from build123d import *

# Parameters (mm, degrees)
F1_DEPTH = 90


with BuildPart() as f1:
    # F0 (on Front) → F1 (new body)
    with BuildSketch(Plane.XZ):
        with BuildLine():
            Line((54.3923101205, -6.9459271067), (39.3923101205, -6.9459271067))
            Line((39.3923101205, -6.9459271067), (24.3923101205, -6.9459271067))
            Line((24.3923101205, -6.9459271067), (24.3923101205, -22.9459271067))
            ThreePointArc((24.3923101205, -22.9459271067), (27.0283490898, -29.3098881374), (33.3923101205, -31.9459271067))
            Line((33.3923101205, -31.9459271067), (39.3923101205, -31.9459271067))
            add(Edge.make_bspline(
                [(54.3923101205, -6.9459271067), (54.7600798309, -12.4650411308), (53.5760512989, -19.2747786322), (51.1416965676, -25.5090219107), (47.6191843875, -29.9359194122), (42.847190561, -31.9967957119), (39.3923101205, -31.9459271067)],
                knots=[0, 0, 0, 0, 0.318087546, 0.5385673182, 0.7419978267, 1, 1, 1, 1], degree=3))
        make_face()
        with BuildLine():
            Line((24.3923101205, -6.9459271067), (39.3923101205, -6.9459271067))
            add(Edge.make_bspline(
                [(39.3923101205, -6.9459271067), (34.4260372221, -4.787703976), (28.490868897, -2.8215542068), (10.9690373288, 1.5413653414), (3.5167664753, 1.7551726321), (0, 1.991873607)],
                knots=[0, 0, 0, 0, 0.3219844291, 0.6966090332, 1, 1, 1, 1], degree=3))
            add(Edge.make_bspline(
                [(-39.3923101205, -6.9459271067), (-34.4260372221, -4.787703976), (-28.490868897, -2.8215542068), (-10.9690373288, 1.5413653414), (-3.5167664753, 1.7551726321), (0, 1.991873607)],
                knots=[0, 0, 0, 0, 0.3219844291, 0.6966090332, 1, 1, 1, 1], degree=3))
            Line((-39.3923101205, -6.9459271067), (-24.3923101205, -6.9459271067))
            add(Edge.make_bspline(
                [(-24.3923101205, -6.9459271067), (-19.7168922052, -5.166058033), (-11.2405807669, -3.1169609653), (-3.7964381143, -2.7464545273), (0, -2.6104990393)],
                knots=[0, 0, 0, 0, 0.5268022864, 1, 1, 1, 1], degree=3))
            add(Edge.make_bspline(
                [(24.3923101205, -6.9459271067), (19.7168922052, -5.166058033), (11.2405807669, -3.1169609653), (3.7964381143, -2.7464545273), (0, -2.6104990393)],
                knots=[0, 0, 0, 0, 0.5268022864, 1, 1, 1, 1], degree=3))
        make_face()
        with BuildLine():
            Line((-24.3923101205, -6.9459271067), (-39.3923101205, -6.9459271067))
            Line((-39.3923101205, -6.9459271067), (-54.3923101205, -6.9459271067))
            add(Edge.make_bspline(
                [(-54.3923101205, -6.9459271067), (-54.7600798309, -12.4650411308), (-53.5760512989, -19.2747786322), (-51.1416965676, -25.5090219107), (-47.6191843875, -29.9359194122), (-42.847190561, -31.9967957119), (-39.3923101205, -31.9459271067)],
                knots=[0, 0, 0, 0, 0.318087546, 0.5385673182, 0.7419978267, 1, 1, 1, 1], degree=3))
            Line((-39.3923101205, -31.9459271067), (-33.3923101205, -31.9459271067))
            ThreePointArc((-33.3923101205, -31.9459271067), (-27.0283490898, -29.3098881374), (-24.3923101205, -22.9459271067))
            Line((-24.3923101205, -22.9459271067), (-24.3923101205, -6.9459271067))
        make_face()
    extrude(amount=F1_DEPTH)


solid = f1.part
Source: CAD feature listing. Evaluate the final solid. Frame: model axes, mm. A direction names the side the tool comes from. Coordinates: 2 decimals unless noted, no trailing zeros.
Item 1: Material intervals for line 1 (Z direction, x = -40.5, y = -10); line 2 (X direction, y = -59.5, z = -30); line 3 (X direction, y = -40, z = -26), sorted ascending.
Output values:
line 1: z = -31.92 to -6.95
line 2: x = -46.57 to -27.8, 27.8 to 46.57
line 3: x = -50.53 to -24.93, 24.93 to 50.53
Item 2: Pull-direction query (X, two-part tool) for faces 1 (the face through (24.392, -44, -15)), 2 (the face through (36, -44, -31.946)); classes: pulls with the +X half, pulls with the -X half, needs draft (parallel to the pull), parting line crosses it, or undercut.
Output values:
face 1: undercut
face 2: needs draft
Item 3: Set-up query: faces 3 (the face through (-47, -44, -6.946)), 4 (the face through (47, -44, -6.946)), 5 (the face through (26.96, -44.37, -29.24)), 6 (the face through (-13, -90, -3)). Return all of +Z, -Z, +X, -X, +Y, -Y with unobstructed straight access to the full face (end or side cutting, diameter ignored); none if empty.
Output values:
face 3: +Z, -X, +Y, -Y
face 4: +Z, +X, +Y, -Y
face 5: -Z, +Y, -Y
face 6: +Z, -Z, +X, -X, -Y
Item 4: First-contact query: P1, Ø4, axis at x = 16.5, y = -59.5, coming from the +Z side; P2, Ø13, axis at y = -64.5, z = -12.5, coming from the -X side; P3, Ø8, axis at x = -25.5, y = -14, coming from the +Z side. Flat tips, straight axial feed; report the tip coordinate or a pass-through.
Output values:
P1: stops at z = 0.41
P2: stops at x = -54.49
P3: stops at z = -1.14
